from build123d import *

# Parameters (mm, degrees)
F0_R      = 25.4
F1_DEPTH  = 19.05
F2_R      = 25.4
F2_R_2    = 22.225
F3_DEPTH  = 3.175
F4_R      = 2.38125
F5_DEPTH  = 63.5
F6_R      = 2.9763912457
F6_R_2    = 2.38125
F7_DEPTH  = 3.175
F8_R      = 22.6060003042
F9_DEPTH  = 3.175
F10_R     = 6.35
F11_DEPTH = 25.4


with BuildPart() as f1:
    # F0 (on Top) → F1 (new body)
    with BuildSketch(Plane.XY):
        Circle(F0_R)
    extrude(amount=F1_DEPTH)

    # F2 (on face) → F3 (join)
    with BuildSketch(Plane.XY.offset(19.05)):
        Circle(F2_R)
        Circle(F2_R_2, mode=Mode.SUBTRACT)
    extrude(amount=-F3_DEPTH)

    # F4 (on Front) → F5 (join)
    with BuildSketch(Plane.XZ):
        with Locations((0, 6.35)):
            Circle(F4_R)
    extrude(amount=F5_DEPTH)

    # F6 (on face) → F7 (join)
    with BuildSketch(Plane.XZ.offset(63.5)):
        with Locations((0, 6.35)):
            Circle(F6_R)
        with Locations((0, 6.35)):
            Circle(F6_R_2, mode=Mode.SUBTRACT)
        with Locations((0, 6.35)):
            Circle(F6_R_2)
    extrude(amount=F7_DEPTH)

    # F8 (on face) → F9 (join)
    with BuildSketch(Plane.XY.offset(19.05)):
        Circle(F8_R)
    extrude(amount=-F9_DEPTH)

    # F10 (on face) → F11 (join)
    with BuildSketch(Plane(origin=(0, 0, 0), x_dir=(1, 0, 0), z_dir=(0, 0, -1))):
        Circle(F10_R)
    extrude(amount=F11_DEPTH)


solid = f1.part
Could you check a few things on this model? Use its own coordinates, in mm. A direction names the side the tool comes from. Round coordinates to 2 decimals unless told otherwise and drop trailing zeros. Order: outer loops, then holes, each group sorted by start corner. A loop starts at its lowest first (then second) coordinate and runs counter-clockwise, first axis right, second up.
(1) I'm going to push flat-ended pins straight in: pin 1 (1 mm diameter, centred on x = -0.5, z = 10, fed in from -Y); pin 2 (10 mm diameter, centred on x = 4, z = -12.5, fed in from +Y); pin 3 (6 mm diameter, centred on y = -31.5, z = 9.5, fed in from +X). Where does each tip first touch, or does it pass through?
Response values:
pin 1: stops at y = -25.4
pin 2: stops at y = 6.35
pin 3: stops at x = 2.38
(2) Imagine slicing it at D-D (z = -13.5). Write out the boundary of the cut face in (x, y), plus the area to 3 significant figures.
Response values:
outline: circle Ø12.7 at (0, 0)
area: 127 mm2
(3) Which directions (+Z, -Z, +X, -X, +Y, -Y) give clear straight access to the entire face, cutting with the end or side of a thin tool? Please do faces 5 (the flat face through (0, 0, 19.05)), 6 (the flat face through (0, -63.5, 9)), 7 (the flat face through (5, -5, 0)).
Response values:
face 5: +Z, +X, -X, +Y, -Y
face 6: none
face 7: -Z
(4) Imagine slicing it at B-B (z = 6.35). Write out the boundary of the cut face in (x, y) (3 decimals), plus the area to 3 significant figures.
Response values:
outline: (-2.976, -66.675) - (2.976, -66.675) - (2.976, -63.5) - (2.381, -63.5) - (2.381, -25.288) arc R25.4 ccw (long way) to (-2.381, -25.288) - (-2.381, -63.5) - (-2.976, -63.5) - close
area: 2,230 mm2
(5) Imagine slicing it at A-A (y = 0). Write out the boundary of the cut face in (x, z), plus the area to 3 significant figures.
Response values:
outline: (-25.4, 0) - (-6.35, 0) - (-6.35, -25.4) - (6.35, -25.4) - (6.35, 0) - (25.4, 0) - (25.4, 19.05) - (-25.4, 19.05) - close
area: 1,290 mm2
(6) Please list where these lines run through material, in increasing order: line 1 along Z through (x, y) = (-13.5, -7.5); line 2 along Y through (x, z) = (5, -4); line 3 along X through (y, z) = (-1.5, -9.5).
Response values:
line 1: z = 0 to 19.05
line 2: y = -3.91 to 3.91
line 3: x = -6.17 to 6.17
(7) Imagine slicing it at C-C (x = 0). Write out the boundary of the cut face in (y, z) (3 decimals).
Response values:
outline: (-66.675, 3.374) - (-63.5, 3.374) - (-63.5, 3.969) - (-25.4, 3.969) - (-25.4, 0) - (-6.35, 0) - (-6.35, -25.4) - (6.35, -25.4) - (6.35, 0) - (25.4, 0) - (25.4, 19.05) - (-25.4, 19.05) - (-25.4, 8.731) - (-63.5, 8.731) - (-63.5, 9.326) - (-66.675, 9.326) - close
(8) If we mould it in two halves opening along Y, with no side actions, what happens to faces 1 (the cylindrical face through (-1.38, 6.2, -12.52)), 2 (the flat face through (0, -66.675, 6)), 3 (the cylindrical face through (-0.645, -65.065, 3.444)), 4 (the cylindrical face through (-0.516, -44.125, 4.025))? For each: released by +Y, released by -Y, zero draft, split by the parting line, or undercut.
Response values:
face 1: split by the parting line
face 2: released by -Y
face 3: zero draft
face 4: undercut
